Geometry check sheet. Reference: the model listing, model coordinates, mm. A direction names the side the tool comes from. Round coordinates to 2 decimals unless told otherwise and drop trailing zeros. Loops run counter-clockwise (first coordinate to the right, second up) from the corner with the lowest first, then second, coordinate; pieces in that order, holes last. Notation, with made-up numbers: M -12,14.5 L 28,14.5 A21 ccw 28,49.5 Z; hole C -40,65 d3. An arc over 180 degrees is marked long. Write item = value, one per line.
from build123d import *

# Parameters (mm, degrees)
SKETCH_1_W          = 24
SKETCH_1_H          = 17
EXTRUDE_1_DEPTH     = 37
CUT_EXTRUDE_1_DEPTH = 15.5
CUT_EXTRUDE_2_REACH = 49.265
SKETCH_3_R          = 0.6
CUT_EXTRUDE_3_REACH = 49.265
SKETCH_4_R          = 0.6
SKETCH_5_W          = 20
SKETCH_5_H          = 2
CUT_EXTRUDE_4_DEPTH = 11
SKETCH_6_W          = 15
SKETCH_6_H          = 1.5
CUT_EXTRUDE_5_DEPTH = 15


with BuildPart() as part:
    # 草图1 → 凸台-拉伸1 (new body)
    with BuildSketch(Plane.XY):
        with Locations((12, 8.5)):
            Rectangle(SKETCH_1_W, SKETCH_1_H)
    extrude(amount=EXTRUDE_1_DEPTH)

    # 草图2 → 切除-拉伸1 (cut)
    with BuildSketch(Plane.XZ):
        Polygon((24, 34.5), (0, 34.5), (0, 18.5), (0, 2.5), (24, 2.5), align=None)
    extrude(amount=-CUT_EXTRUDE_1_DEPTH, mode=Mode.SUBTRACT)

    # 草图3 → 切除-拉伸2 (cut, up to next)
    with BuildSketch(Plane.XY.offset(37), mode=Mode.PRIVATE) as cut_extrude_2_sk1:
        with Locations((1.75, 9.2)):
            Circle(SKETCH_3_R)
    cut_extrude_2_tool1 = extrude(cut_extrude_2_sk1.sketch, amount=-CUT_EXTRUDE_2_REACH, mode=Mode.PRIVATE) & part.part
    # 草图3 → 切除-拉伸2 (cut, up to next)
    with BuildSketch(Plane.XY.offset(37), mode=Mode.PRIVATE) as cut_extrude_2_sk2:
        with Locations((22.25, 9.2)):
            Circle(SKETCH_3_R)
    cut_extrude_2_tool2 = extrude(cut_extrude_2_sk2.sketch, amount=-CUT_EXTRUDE_2_REACH, mode=Mode.PRIVATE) & part.part
    add(cut_extrude_2_tool1.solids().sort_by_distance((1.75, 9.2, 37))[0], mode=Mode.SUBTRACT)
    add(cut_extrude_2_tool2.solids().sort_by_distance((22.25, 9.2, 37))[0], mode=Mode.SUBTRACT)

    # 草图4 → 切除-拉伸3 (cut, up to next)
    with BuildSketch(Plane(origin=(0, 0, 0), x_dir=(-1, 0, 0), z_dir=(0, 0, -1)), mode=Mode.PRIVATE) as cut_extrude_3_sk1:
        with Locations((-22.25, 12.95)):
            Circle(SKETCH_4_R)
    cut_extrude_3_tool1 = extrude(cut_extrude_3_sk1.sketch, amount=-CUT_EXTRUDE_3_REACH, mode=Mode.PRIVATE) & part.part
    # 草图4 → 切除-拉伸3 (cut, up to next)
    with BuildSketch(Plane(origin=(0, 0, 0), x_dir=(-1, 0, 0), z_dir=(0, 0, -1)), mode=Mode.PRIVATE) as cut_extrude_3_sk2:
        with Locations((-1.75, 12.95)):
            Circle(SKETCH_4_R)
    cut_extrude_3_tool2 = extrude(cut_extrude_3_sk2.sketch, amount=-CUT_EXTRUDE_3_REACH, mode=Mode.PRIVATE) & part.part
    add(cut_extrude_3_tool1.solids().sort_by_distance((22.25, 12.95, 0))[0], mode=Mode.SUBTRACT)
    add(cut_extrude_3_tool2.solids().sort_by_distance((1.75, 12.95, 0))[0], mode=Mode.SUBTRACT)

    # 草图5 → 切除-拉伸4 (cut)
    with BuildSketch(Plane.XZ):
        with Locations((12, 1.5)):
            Rectangle(SKETCH_5_W, SKETCH_5_H)
    extrude(amount=-CUT_EXTRUDE_4_DEPTH, mode=Mode.SUBTRACT)

    # 草图6 → 切除-拉伸5 (cut)
    with BuildSketch(Plane.XZ):
        with Locations((12, 35.25)):
            Rectangle(SKETCH_6_W, SKETCH_6_H)
    extrude(amount=-CUT_EXTRUDE_5_DEPTH, mode=Mode.SUBTRACT)

    # 镜向1: part across plane


with BuildPart() as part_1:
    add(part.part)
    add(part.part.mirror(Plane.ZX.offset(17)))


solid = part_1.part
(1) Depth check by flat-ended pin: pin 1 Ø1.2 at (x, z) = (9.5, 35) entering from +Y; pin 2 Ø8 at (x, z) = (7, 20.5) entering from +Y; pin 3 Ø1.1 at (x, y) = (22.25, 24.8) entering from +Z. Enter the tip coordinate at first touch or a pass-through.
Result set:
pin_1 = 19
pin_2 = 18.5
pin_3 = 2.5
(2) Tool access check on faces 1 (the flat face through (12, 27, 36)), 2 (the flat face through (12, 13, 2.5)), 3 (the cylindrical face through (21.678, 13.13, 1.232)), 4 (the flat face through (19.5, 7, 35)). Record the directions out of +Z, -Z, +X, -X, +Y, -Y that give a thin tool (end or side, any length) a straight path to the whole face; none if there is none.
Result set:
face_1 = +Y
face_2 = +X, -X, -Y
face_3 = -Z
face_4 = -Y
(3) Sectioned sample at C-C on x = 10.5. Record the cut outline in (y, z).
Result set:
outline = M 0,0 L 34,0 L 34,0.5 L 23,0.5 L 23,2.5 L 18.5,2.5 L 18.5,34.5 L 19,34.5 L 19,36 L 34,36 L 34,37 L 0,37 L 0,36 L 15,36 L 15,34.5 L 15.5,34.5 L 15.5,2.5 L 11,2.5 L 11,0.5 L 0,0.5 Z
(4) Sectioned sample at A-A on y = 23.5. Record the cut outline in (x, z).
Result set:
outline = M 0,0 L 24,0 L 24,2.5 L 22,2.5 L 22,0.5 L 2,0.5 L 2,2.5 L 0,2.5 Z; M 0,34.5 L 4.5,34.5 L 4.5,36 L 19.5,36 L 19.5,34.5 L 24,34.5 L 24,37 L 0,37 Z
(5) Release check for a two-part mould opening along X. For faces 5 (the flat face through (11.8, 34, 36.3)), 6 (the flat face through (24, 17, 18)), 7 (the flat face through (22, 5, 1)) record: released by +X, released by -X, zero draft, split by the parting line, or undercut.
Result set:
face_5 = zero draft
face_6 = released by +X
face_7 = undercut
(6) Sectioned sample at B-B on y = 12.95. Record the cut outline in (x, z), then the cut area to 3 significant figures.
Result set:
outline = M 0,0 L 1.15,0 L 1.15,2.5 L 0,2.5 Z; M 0,34.5 L 4.5,34.5 L 4.5,36 L 19.5,36 L 19.5,34.5 L 24,34.5 L 24,37 L 0,37 Z; M 2.35,0 L 21.65,0 L 21.65,2.5 L 2.35,2.5 Z; M 22.85,0 L 24,0 L 24,2.5 L 22.85,2.5 Z
area = 91.5 mm2
(7) Material ranges on line 1 along Y through (x, z) = (22.25, 35.3); line 2 along X through (y, z) = (21.05, 1); line 3 along Y through (x, z) = (1.75, 1.45), recorded low to high. Write a range as from..to.
Result set:
line_1 = 0..8.6, 9.8..24.2, 25.4..34
line_2 = 0..1.15, 2.35..21.65, 22.85..24
line_3 = 0..12.35, 13.55..20.45, 21.65..34
(8) Sectioned sample at D-D on y = 20. Record the cut outline in (x, z).
Result set:
outline = M 0,0 L 24,0 L 24,2.5 L 0,2.5 Z; M 0,34.5 L 4.5,34.5 L 4.5,36 L 19.5,36 L 19.5,34.5 L 24,34.5 L 24,37 L 0,37 Z
